from build123d import *

# Parameters (mm, degrees)
F0_W     = 50
F0_H     = 50
F1_DEPTH = 50
F3_DEPTH = 25


with BuildPart() as f1:
    # F0 (on Top) → F1 (new body)
    with BuildSketch(Plane.XY):
        Rectangle(F0_W, F0_H)
    extrude(amount=F1_DEPTH)

    # F2 (on face) → F3 (cut)
    with BuildSketch(Plane.XZ.offset(25)):
        with BuildLine():
            ThreePointArc((4.058878, 12.877418), (9.22055, 16.980929), (11.167368, 23.281053))
            ThreePointArc((11.167368, 23.281053), (-6.300124, 32.501603), (-4.058878, 12.877418))
            ThreePointArc((-4.058878, 12.877418), (0, 12.498873), (4.058878, 12.877418))
        make_face()
    extrude(amount=-F3_DEPTH, mode=Mode.SUBTRACT)


solid = f1.part
Design review of the part built by this model. Coordinates are the model's own, in mm. A direction names the side the tool comes from. Coordinates: 2 decimals unless noted, no trailing zeros. Order: outer loops, then holes, each group sorted by start corner. A loop starts at its lowest first (then second) coordinate and runs counter-clockwise, first axis right, second up.
Item 1: Take a section at C-C, the plane z = 19. Write out the cut boundary in (x, y), then the cut area to 3 significant figures.
Item 2: For faces 5 (the cylindrical face through (-0.1, -12.7, 12.5)), 6 (the flat face through (-25, 0, 25)), list the 3-axis set-ups (+Z, -Z, +X, -X, +Y, -Y) from which the entire face can be reached by the end or side of a thin tool; tool diameter is ignored.
Item 3: Take a section at A-A, the plane y = -19. Write out the cut boundary in (x, z), then the cut area to 3 significant figures.
Item 4: The part is to be moulded in two halves that separate along Z. For faces 1 (the flat face through (0, 0, 50)), 2 (the flat face through (0, 0, 24)), 3 (the flat face through (0, 0, 0)), 4 (the flat face through (0, 25, 25)), say which applies: pulls with the +Z half, pulls with the -Z half, needs draft (parallel to the pull), parting line crosses it, or undercut.
Item 5: For pin 1 Ø13.5 at (x, z) = (0, 23.28) entering from -Y, flat-tipped, find the tip position at first contact; note if it passes through.
Item 6: Take a section at B-B, the plane x = 0. Write out the cut boundary in (y, z), then the cut area to 3 significant figures.
Item 7: For line 1 (Z direction, x = 0, y = -13); line 2 (Z direction, x = -5, y = -4.5); line 3 (Y direction, x = 2, z = 25), list the stretches that pass through material, from the lowest coordinate up.
The answers:
1. outline: (-25, -25) - (-10.31, -25) - (-10.31, 0) - (10.31, 0) - (10.31, -25) - (25, -25) - (25, 25) - (-25, 25) - close
1. area: 1,980 mm2
2. face 5: -Y
2. face 6: +Z, -Z, -X, +Y, -Y
3. outline: (-25, 0) - (25, 0) - (25, 50) - (-25, 50) - close; hole (-4.06, 12.88) arc R21.95 ccw to (4.06, 12.88) arc R11.17 ccw to (11.17, 23.28) arc R11.17 ccw (long way) to start
3. area: 2,110 mm2
4. face 1: pulls with the +Z half
4. face 2: undercut
4. face 3: pulls with the -Z half
4. face 4: needs draft
5. pin 1: stops at y = 0
6. outline: (-25, 0) - (25, 0) - (25, 50) - (-25, 50) - (-25, 34.45) - (0, 34.45) - (0, 12.5) - (-25, 12.5) - close
6. area: 1,950 mm2
7. line 1: z = 0 to 12.5, 34.45 to 50
7. line 2: z = 0 to 13.3, 33.27 to 50
7. line 3: y = 0 to 25
